Study the drawing (mm; zero at the part's minimum x, y, z) and answer. Coordinates: 2 decimals unless noted, no trailing zeros. Loops run counter-clockwise (first coordinate to the right, second up) from the corner with the lowest first, then second, coordinate; pieces in that order, holes last. Notation, with made-up numbers: (-19.75, 49) - (-8.75, 49) arc R21 ccw to (-8.75, 86) - close; hole circle Ø9 at (-30.75, 28). An arc over 180 degrees is marked (long way). Use one line per item in the form item = value.
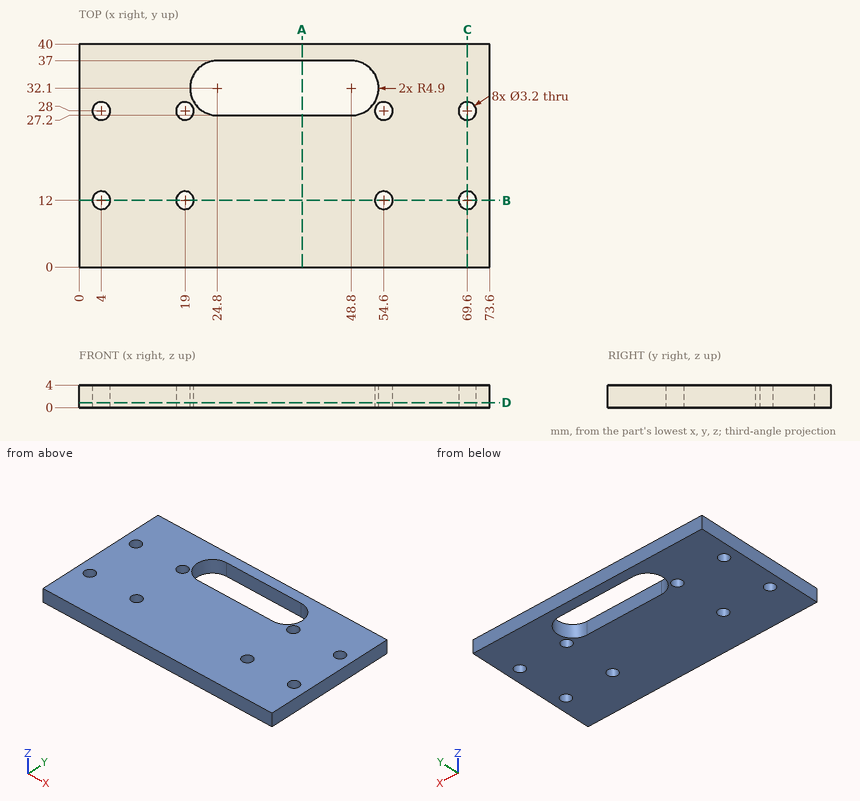
Item 1: Find the intervals of material crossed by L1, parallel to Y at x = 4, z = 2.65; L2, parallel to X at y = 32, z = 3.3; L3, parallel to Y at x = 49, z = 1.9, in increasing order.
Results below:
L1 = 0 to 10.4, 13.6 to 26.4, 29.6 to 40
L2 = 0 to 19.9, 53.7 to 73.6
L3 = 0 to 27.2, 37 to 40
Item 2: The part is cut by section B-B on y = 12. Give the vertices of the cut face in (x, z), plus the area to 3 significant figures.
Results below:
outline = (0, 0) - (2.4, 0) - (2.4, 4) - (0, 4) - close; (5.6, 0) - (17.4, 0) - (17.4, 4) - (5.6, 4) - close; (20.6, 0) - (53, 0) - (53, 4) - (20.6, 4) - close; (56.2, 0) - (68, 0) - (68, 4) - (56.2, 4) - close; (71.2, 0) - (73.6, 0) - (73.6, 4) - (71.2, 4) - close
area = 243 mm²
Item 3: The part is cut by section A-A on x = 40. Give the vertices of the cut face in (y, z).
Results below:
outline = (0, 0) - (27.2, 0) - (27.2, 4) - (0, 4) - close; (37, 0) - (40, 0) - (40, 4) - (37, 4) - close
Item 4: This flat-tipped pin is pushed along its axis until it touches: P1, Ø1.9, axis at x = 54.6, y = 28, coming from the -Z side. Where does it stop, or does it pass through?
Results below:
P1 = through
Item 5: The part is cut by section D-D on z = 0.9. Count the separate pieces of the cut face and the enclosed holes in it, plus the area to 3 significant figures.
Results below:
separate_pieces = 1
enclosed_holes = 9
area = 2,570 mm²
Item 6: The part is cut by section C-C on x = 69.6. Give the vertices of the cut face in (y, z), plus the area to 3 significant figures.
Results below:
outline = (0, 0) - (10.4, 0) - (10.4, 4) - (0, 4) - close; (13.6, 0) - (26.4, 0) - (26.4, 4) - (13.6, 4) - close; (29.6, 0) - (40, 0) - (40, 4) - (29.6, 4) - close
area = 134 mm²
